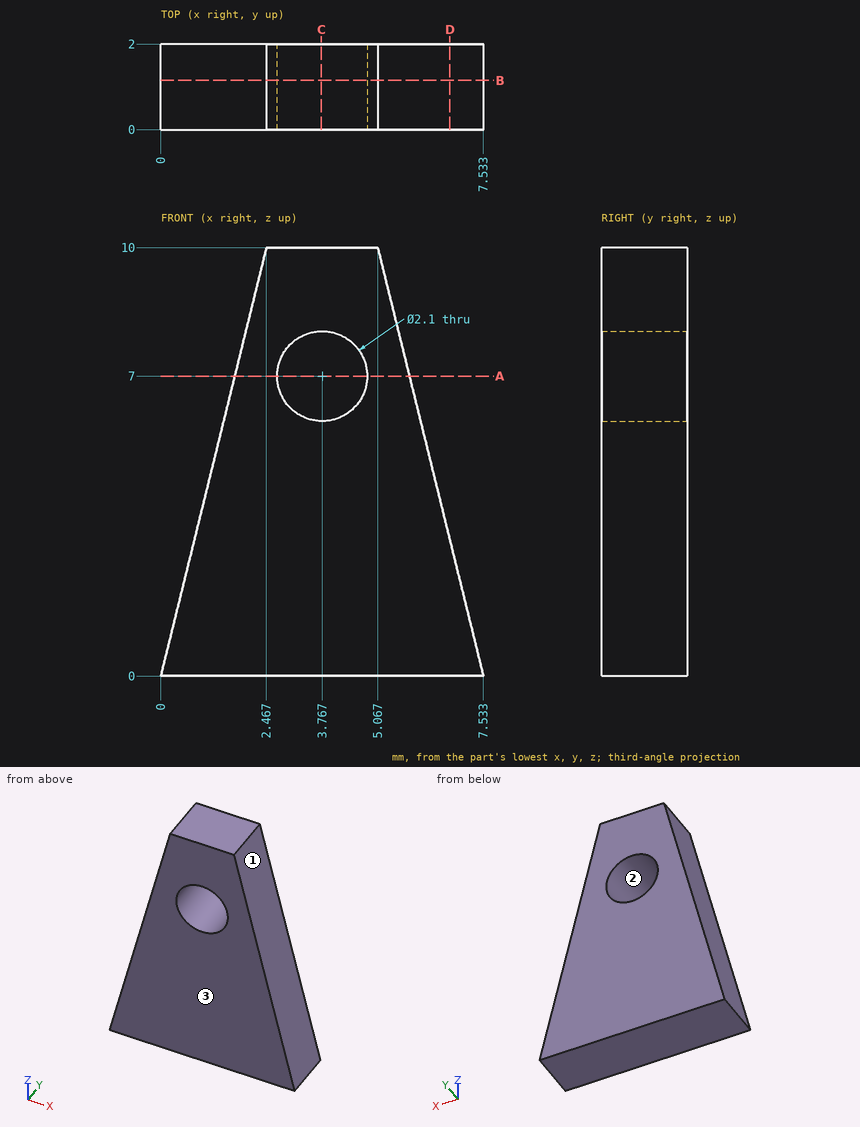
Here's the drawing with two shaded views (mm, measured from the low corner). I have some questions. Give positions to 0.01 mm unless a question says otherwise; leave off trailing zeros. Write each loop counter-clockwise with the first axis right and the second up, starting at its lowest first coordinate (ties: lowest second). Pieces come first, ordered by that corner, then holes. Notation, with made-up numbers: (-14, 37.5) - (20, 37.5) arc R22 ccw to (20, 45.5) - close; hole circle Ø5 at (50, -28.75). An arc over 180 degrees is marked (long way). One line per item, written item: value. Start each with the question number.
Item 1: Imagine slicing it at D-D, the plane x = 6.75. List the corners of the cut face in (y, z) for me (1 decimal).
Item 2: I'm going to push a flat-ended pin straight in: pin 1 (1.9 mm diameter, centred on x = 3.77, z = 7, fed in from -Y). Where does the tip first touch, or does it pass through?
Item 3: Imagine slicing it at C-C, the plane x = 3.75. List the corners of the cut face in (y, z) for me, and give its area (3 significant figures).
Item 4: Imagine slicing it at B-B, the plane y = 1.15. List the corners of the cut face in (x, z) for me.
Item 5: Imagine slicing it at A-A, the plane z = 7. List the corners of the cut face in (x, y) for me.
Item 6: Please list where these lines run through material, in increasing order: line 1 (Z direction, x = 3.75, y = 0.4); line 2 (Z direction, x = 3, y = 0.7); line 3 (X direction, y = 1.3, z = 1.5). Write a range as from..to.
Item 7: If we mould it in two halves opening along X, with no side actions, what happens to the marked faces 1, 2 and 3? For each: +X half, -X half, draft (parallel to the pull), parting line (faces both ways), or undercut.
Geometry says:
1. outline: (0, 0) - (2, 0) - (2, 3.2) - (0, 3.2) - close
2. pin 1: through
3. outline: (0, 0) - (2, 0) - (2, 5.95) - (0, 5.95) - close; (0, 8.05) - (2, 8.05) - (2, 10) - (0, 10) - close
3. area: 15.8 mm^2
4. outline: (0, 0) - (7.53, 0) - (5.07, 10) - (2.47, 10) - close; hole circle Ø2.1 at (3.77, 7)
5. outline: (1.73, 0) - (2.72, 0) - (2.72, 2) - (1.73, 2) - close; (4.82, 0) - (5.81, 0) - (5.81, 2) - (4.82, 2) - close
6. line 1: 0..5.95, 8.05..10
6. line 2: 0..6.28, 7.72..10
6. line 3: 0.37..7.16
7. face 1: +X half
7. face 2: undercut
7. face 3: draft
